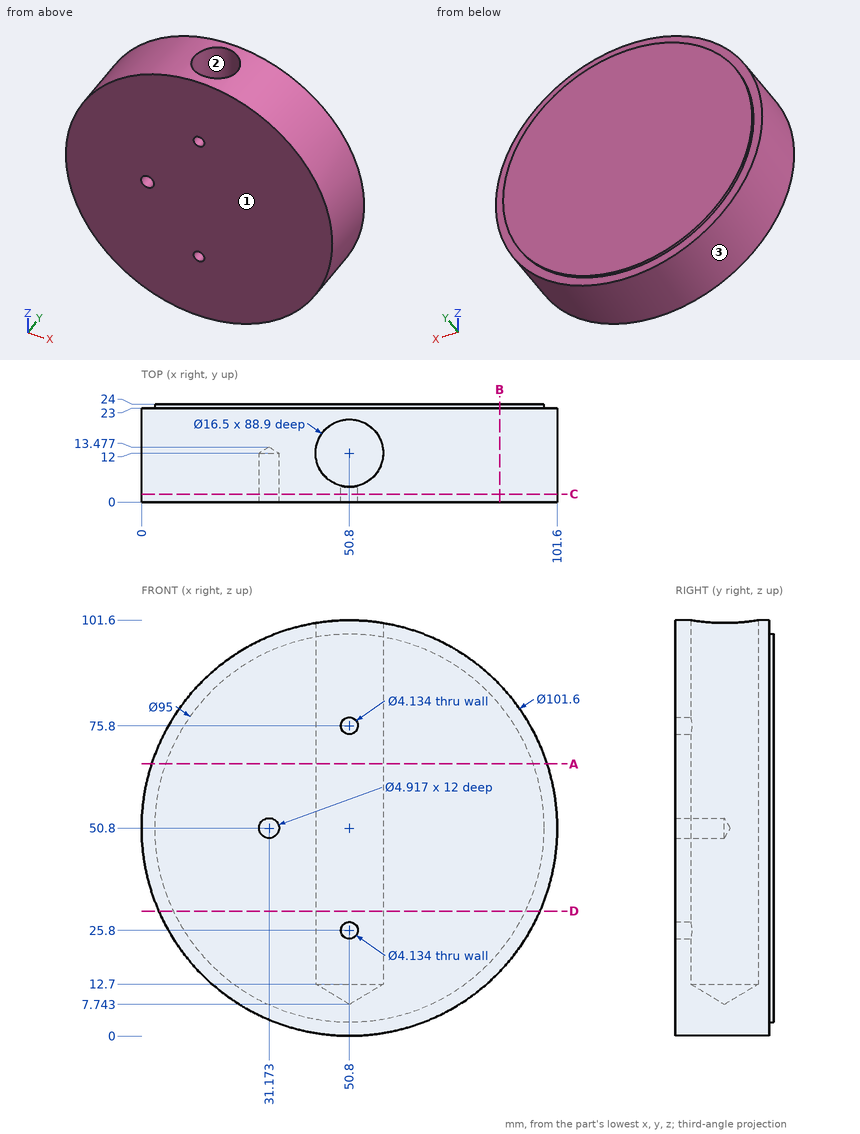
Can you work these out from the drawing? Everything is in mm from the part's minimum corner. Round coordinates to 2 decimals unless told otherwise and drop trailing zeros. Write each loop counter-clockwise with the first axis right and the second up, starting at its lowest first coordinate (ties: lowest second). Pieces come first, ordered by that corner, then holes.
1. I need wall thicknesses on L1, parallel to X at y = 2.35, z = 75.8; L2, parallel to X at y = 12, z = 73; L3, parallel to Y at x = 50, z = 51. Which ranges of each line are inside material? Lowest first, please.
2. If we mould it in two halves opening along X, with no side actions, what happens to the marked faces 1, 2 and 3? For each: released by +X, released by -X, zero draft, split by the parting line, or undercut.
3. Suppose I cut it at D-D (z = 30.5). List the corners of the cut face in (x, y) for me, and give its area (3 significant figures).
4. Suppose I cut it at A-A (z = 66.5). List the corners of the cut face in (x, y) for me.
5. Suppose I cut it at B-B (x = 87.5). List the corners of the cut face in (y, z) for me (1 decimal).
6. Suppose I cut it at C-C (y = 2). List the corners of the cut face in (x, z) for me.
7. Will these pins go through, and if not, where does the flat tip stop? pin 1 Ø4 at (y, z) = (3, 56) entering from +X; pin 2 Ø6 at (x, y) = (54.5, 14) entering from -Z (3 decimals); pin 3 Ø2.5 at (x, z) = (50.8, 25.8) entering from -Y (1 decimal).
Answer sheet:
1. L1: x = 6.58 to 48.73, 52.87 to 95.02
1. L2: x = 5.11 to 42.55, 59.05 to 96.49
1. L3: y = 0 to 3.79, 20.21 to 24
2. face 1: zero draft
2. face 2: undercut
2. face 3: split by the parting line
3. outline: (4.23, 0) - (97.37, 0) - (97.37, 23) - (93.74, 23) - (93.74, 24) - (7.86, 24) - (7.86, 23) - (4.23, 23) - close; hole circle Ø16.5 at (50.8, 12)
3. area: 2,010 mm2
4. outline: (2.49, 0) - (99.11, 0) - (99.11, 23) - (95.63, 23) - (95.63, 24) - (5.97, 24) - (5.97, 23) - (2.49, 23) - close; hole circle Ø16.5 at (50.8, 12)
5. outline: (0, 15.7) - (23, 15.7) - (23, 20.6) - (24, 20.6) - (24, 81) - (23, 81) - (23, 85.9) - (0, 85.9) - close
6. outline: circle Ø101.6 at (50.8, 50.8); hole circle Ø4.92 at (31.17, 50.8); hole circle Ø4.13 at (50.8, 25.8); hole circle Ø4.13 at (50.8, 75.8)
7. pin 1: stops at x = 101.5
7. pin 2: stops at z = 0.005
7. pin 3: stops at y = 20.2
